Study the drawing (mm; zero at the part's minimum x, y, z) and answer. A direction names the side the tool comes from. Round coordinates to 2 decimals unless told otherwise and drop trailing zeros. Loops run counter-clockwise (first coordinate to the right, second up) from the corner with the lowest first, then second, coordinate; pieces in that order, holes last. Notation, with made-up numbers: (61.25, -24) - (87.25, -24) arc R17 cw to (87.25, -10) - close; hole circle Ø10 at (-31.75, 80.5). An arc over 180 degrees is marked (long way). One line per item, written item: value.
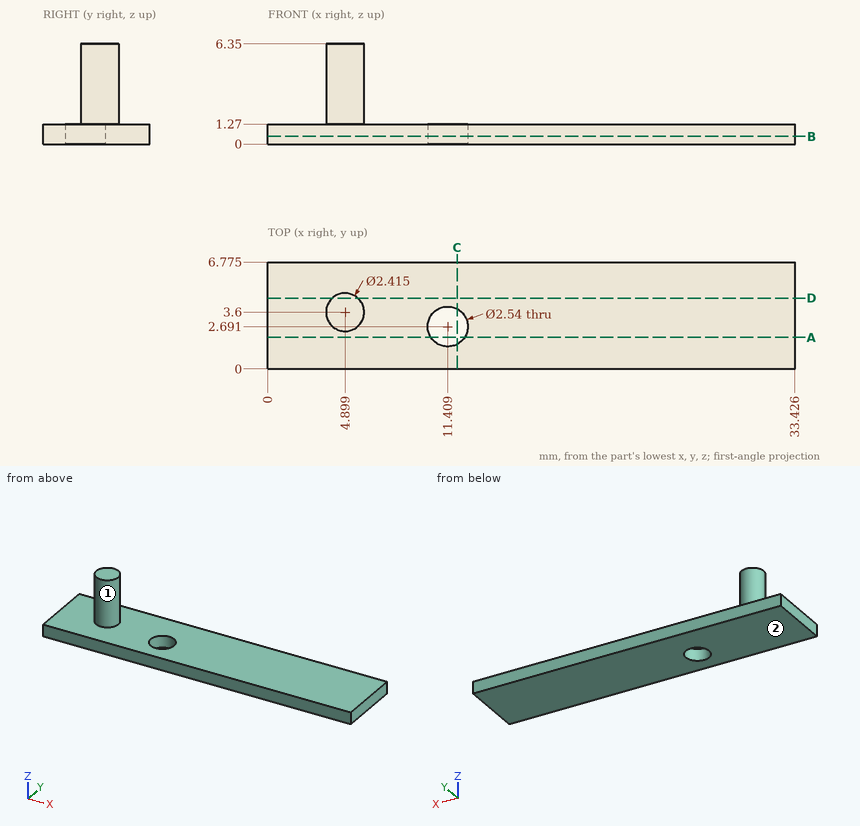
1) A cutting plane is placed at A-A on y = 2. Give the vertices of the cut face in (x, z) (1 decimal).
Final values:
outline: (0, 0) - (10.3, 0) - (10.3, 1.3) - (0, 1.3) - close; (12.5, 0) - (33.4, 0) - (33.4, 1.3) - (12.5, 1.3) - close
2) A cutting plane is placed at C-C on x = 12. Give the vertices of the cut face in (y, z) (1 decimal).
Final values:
outline: (0, 0) - (1.6, 0) - (1.6, 1.3) - (0, 1.3) - close; (3.8, 0) - (6.8, 0) - (6.8, 1.3) - (3.8, 1.3) - close
3) For the marked faces 1 and 2, determine the directions among +Z, -Z, +X, -X, +Y, -Y from which every point of the face is accessible in a straight line to the end or side of a thin tool.
Final values:
face 1: +Z
face 2: -Z, +X, -X, +Y, -Y
4) Consider L1, parallel to Z at x = 31, y = 0.5; L2, parallel to X at y = 4.25, z = 3.25 (1 decimal); L3, parallel to X at y = 3.75, z = 2.5. Determine where each line is inside the solid, lowest interval first.
Final values:
L1: 0 to 1.27
L2: 3.9 to 5.9
L3: 3.7 to 6.1
5) Each of these flat-tipped pins is pushed along its axis until it touches: pin 1 Ø3.5 at (x, y) = (21, 3.5) entering from +Z; pin 2 Ø1.5 at (x, y) = (26.5, 3) entering from -Z; pin 3 Ø1.5 at (y, z) = (4.5, 2.5) entering from +X. Where does it stop, or does it pass through?
Final values:
pin 1: z = 1.27
pin 2: z = 0
pin 3: x = 6.1
6) A cutting plane is placed at D-D on y = 4.5. Give the vertices of the cut face in (x, z).
Final values:
outline: (0, 0) - (33.43, 0) - (33.43, 1.27) - (5.7, 1.27) - (5.7, 6.35) - (4.09, 6.35) - (4.09, 1.27) - (0, 1.27) - close
7) A cutting plane is placed at B-B on z = 0.5. Give the vertices of the cut face in (x, y) (1 decimal), and give its area (3 significant figures).
Final values:
outline: (0, 0) - (33.4, 0) - (33.4, 6.8) - (0, 6.8) - close; hole circle Ø2.5 at (11.4, 2.7)
area: 221 mm2
